Can you work these out from the model? Positions are in its coordinate system, mm. A direction names the side the tool comes from. Give positions to 0.01 mm unless a question says otherwise; leave off trailing zeros. Write each loop counter-clockwise with the first axis right and the second up, starting at its lowest first coordinate (ties: lowest second). Pieces come first, ordered by that corner, then holes. Notation, with made-up numbers: M -10.5,47.5 L 30.5,47.5 A20 cw 30.5,84.5 Z; hole C -16,-31.75 d1. An arc over 180 degrees is marked long. Write each question's results on one line, items separated by ' | '.
from build123d import *

# Parameters (mm, degrees)
PAD_DEPTH       = 25
POCKET_DEPTH    = 23
SKETCH002_R     = 8.25
POCKET001_DEPTH = 25


with BuildPart() as part:
    # Sketch → Pad (new body)
    with BuildSketch(Plane.XY):
        with BuildLine():
            Line((-13, 0), (-13, 13))
            Line((-13, 13), (13, 13))
            Line((13, 13), (13, 0))
            ThreePointArc((-13, 0), (0, -13), (13, 0))
        make_face()
    extrude(amount=PAD_DEPTH)

    # Sketch001 (on DatumPlane) → Pocket (cut)
    with BuildSketch(Plane.XY.offset(25)):
        with BuildLine():
            Line((-11, 0), (-11, 11))
            Line((-11, 11), (11, 11))
            Line((11, 11), (11, 0))
            ThreePointArc((-11, 0), (0, -11), (11, 0))
        make_face()
    extrude(amount=-POCKET_DEPTH, mode=Mode.SUBTRACT)

    # Sketch002 (on DatumPlane) → Pocket001 (cut)
    with BuildSketch(Plane.XY.offset(25)):
        Circle(SKETCH002_R)
    extrude(amount=-POCKET001_DEPTH, mode=Mode.SUBTRACT)


solid = part.part
Item 1: I'm going to push flat-ended pins straight in: pin 1 (10 mm diameter, centred on x = 1.5, z = 14, fed in from -Y); pin 2 (10 mm diameter, centred on x = 2.5, y = 2.5, fed in from +Z). Where does each tip first touch, or does it pass through?
Geometry says:
pin 1: stops at y = -13 | pin 2: stops at z = 2
Item 2: I want a section at D-D, the plane y = 9.5. Please give me the cut outline in (x, z), and give its area (3 significant figures).
Geometry says:
outline: M -13,0 L 13,0 L 13,25 L 11,25 L 11,2 L -11,2 L -11,25 L -13,25 Z | area: 144 mm2
Item 3: Thinking about a two-plate mould opening in Y: for faces 3 (the face through (0, 9, 0)), 4 (the face through (0, 13, 12)), 5 (the face through (11, 6, 14)), which applies, +Y half, -Y half, draft (parallel to the pull), parting line (faces both ways), or undercut?
Geometry says:
face 3: draft | face 4: +Y half | face 5: undercut
Item 4: I want a section at A-A, the plane z = 16.75. Please give me the cut outline in (x, y), and give its area (3 significant figures).
Geometry says:
outline: M -13,0 A13 ccw 13,0 L 13,13 L -13,13 Z; hole M -11,0 A11 ccw 11,0 L 11,11 L -11,11 Z | area: 171 mm2
Item 5: For faces 1 (the face through (7.62, -3.16, 1.01)), 2 (the face through (-11, 5, 14)), which set-ups out of +Z, -Z, +X, -X, +Y, -Y let a thin tool reach every point of the face, with its end or its side?
Geometry says:
face 1: +Z, -Z | face 2: +Z
Item 6: If I drill on line 1 (X direction, y = 1.25, z = 20.25); line 2 (Y direction, x = 0, z = 1); line 3 (Y direction, x = 6.25, z = 1.75), over which ranges is the centre line in solid material (lowest first)? Write a range as from..to.
Geometry says:
line 1: x = -13..-11, 11..13 | line 2: y = -13..-8.25, 8.25..13 | line 3: y = -11.4..-5.39, 5.39..13
Item 7: I want a section at C-C, the plane y = 4.25. Please give me the cut outline in (x, z), and give its area (3 significant figures).
Geometry says:
outline: M -13,0 L -7.07,0 L -7.07,2 L -11,2 L -11,25 L -13,25 Z; M 7.07,0 L 13,0 L 13,25 L 11,25 L 11,2 L 7.07,2 Z | area: 116 mm2
Item 8: I want a section at B-B, the plane x = 0. Please give me the cut outline in (y, z), and give its area (3 significant figures).
Geometry says:
outline: M -13,0 L -8.25,0 L -8.25,2 L -11,2 L -11,25 L -13,25 Z; M 8.25,0 L 13,0 L 13,25 L 11,25 L 11,2 L 8.25,2 Z | area: 111 mm2
